Check sheet for the drawn part. Datum: minimum x, y, z corner. Units: mm. Coordinates: 2 decimals unless noted, no trailing zeros. Loops run counter-clockwise (first coordinate to the right, second up) from the corner with the lowest first, then second, coordinate; pieces in that order, holes last.
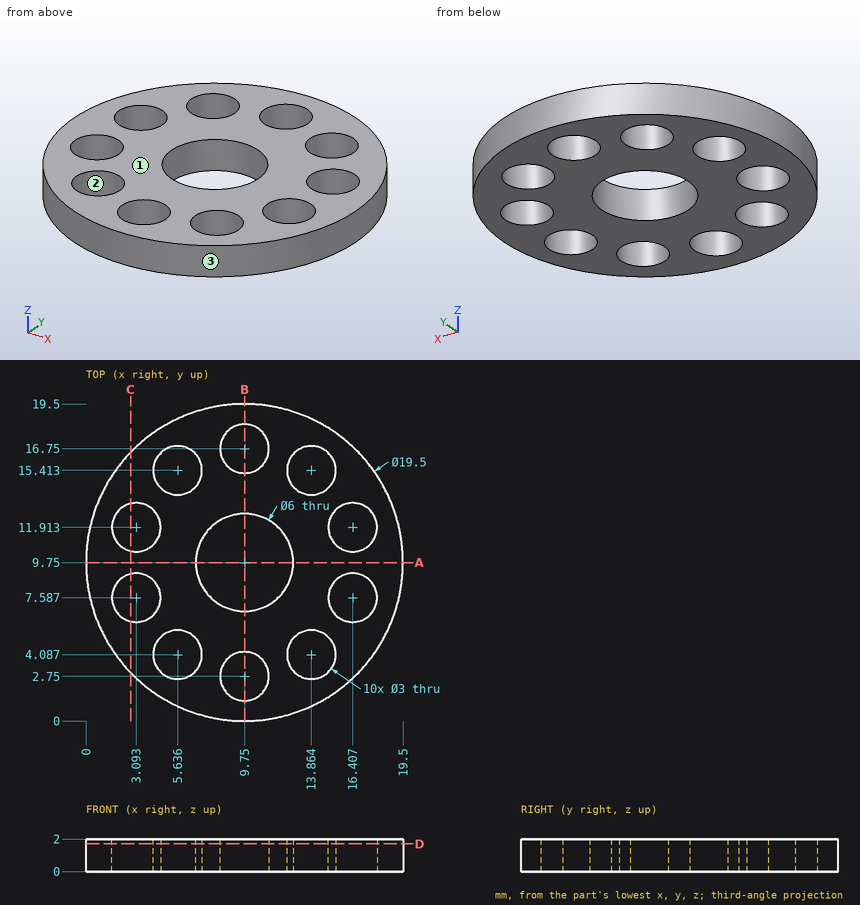
(1) Draft check along Y on the marked faces 1, 2 and 3. Enter one of: +Y half, -Y half, draft (parallel to the pull), parting line (faces both ways), or undercut.
Findings:
face 1: draft
face 2: undercut
face 3: parting line
(2) Sectioned sample at A-A on y = 9.75. Record the cut outline in (x, z).
Findings:
outline: (0, 0) - (6.75, 0) - (6.75, 2) - (0, 2) - close; (12.75, 0) - (19.5, 0) - (19.5, 2) - (12.75, 2) - close
(3) Scan lines: L1, parallel to Y at x = 9.75, z = 0.8; L2, parallel to X at y = 5, z = 1.55 (1 decimal); L3, parallel to X at y = 15, z = 1.6 (1 decimal). Record each from-to range of solid material in increasing order.
Findings:
L1: y = 0 to 1.25, 4.25 to 6.75, 12.75 to 15.25, 18.25 to 19.5
L2: x = 1.2 to 4.4, 6.8 to 12.7, 15.1 to 18.3
L3: x = 1.5 to 4.2, 7.1 to 12.4, 15.3 to 18
(4) Sectioned sample at D-D on z = 1.7. State how many separate pieces and enclosed holes the cut face has, and give its area (3 significant figures).
Findings:
separate pieces: 1
enclosed holes: 11
area: 200 mm2
(5) Gauge pin test, flat end, axial feed: pin 1 Ø2.5 at (x, y) = (13.86, 15.41) entering from +Z. Record the tip position at first contact, or that the pin passes through.
Findings:
pin 1: passes through
(6) Sectioned sample at B-B on x = 9.75. Record the cut outline in (y, z), and give its area (3 significant figures).
Findings:
outline: (0, 0) - (1.25, 0) - (1.25, 2) - (0, 2) - close; (4.25, 0) - (6.75, 0) - (6.75, 2) - (4.25, 2) - close; (12.75, 0) - (15.25, 0) - (15.25, 2) - (12.75, 2) - close; (18.25, 0) - (19.5, 0) - (19.5, 2) - (18.25, 2) - close
area: 15.0 mm2
(7) Sectioned sample at C-C on x = 2.75. Record the cut outline in (y, z).
Findings:
outline: (2.96, 0) - (6.13, 0) - (6.13, 2) - (2.96, 2) - close; (9.05, 0) - (10.45, 0) - (10.45, 2) - (9.05, 2) - close; (13.37, 0) - (16.54, 0) - (16.54, 2) - (13.37, 2) - close
